The listing builds one solid part. Answer for the finished solid, in the listing's coordinates (mm). A direction names the side the tool comes from. Give positions to 0.01 mm unless a question says otherwise; leave off trailing zeros. Loops run counter-clockwise (first coordinate to the right, second up) from the corner with the lowest first, then second, coordinate; pieces in that order, holes last. Notation, with made-up numbers: (22.25, 30.25) - (32.25, 30.25) arc R24 cw to (32.25, 63.25) - close; hole circle Ø8 at (33, 9.5). An arc over 180 degrees is marked (long way). Write item = value, one per line. Start each with the question number.
1) The part is cut by section B-B on y = -5. Write down the section's boundary in (x, z).
2) The mould has two halves that part along Y. Classify faces 1 (the cylindrical face through (-4.385, 2.465, 2.895)), 2 (the flat face through (-6, -5.5, 6)), 3 (the flat face through (-13, 0, 13)): +Y half, -Y half, draft (parallel to the pull), parting line (faces both ways), or undercut.
3) The part is cut by section A-A on x = -21.5. Write down the section's boundary in (y, z).
4) A flat-ended cylindrical pin translates along its axis: P1, Ø1, axis at x = -15, z = 9, coming from the +Y side. Find the tip coordinate at first contact, or state that the pin passes through.
5) The part is cut by section D-D on y = 1.5. Write down the section's boundary in (x, z).
6) Which of the six approach directions +Z, -Z, +X, -X, +Y, -Y give full straight-line access (tool end or side, diameter ignored) to faces 4 (the flat face through (-19, 5, 19)), 5 (the cylindrical face through (-6.46, 2.46, 22.47)), 6 (the flat face through (-20, -5.5, 20))?
7) Consider probe 1 along X at (y, z) = (-3.7, 19.5); probe 2 along Z at (x, y) = (-19.5, -3.45); probe 3 along Y at (x, z) = (-19, 17.5). Determine where each line is inside the solid, lowest interval first.
8) The part is cut by section C-C on z = 21.75. Write down the section's boundary in (x, y), plus the area to 3 significant figures.
from build123d import *

# Parameters (mm, degrees)
F0_W      = 25
F0_H      = 25
F1_DEPTH  = 10
F2_R      = 3.5
F3_DEPTH  = 5
F4_R      = 4
F1_FACE_W = 25
F1_FACE_H = 25
F5_DEPTH  = 5.5


with BuildPart() as f1:
    # F0 (on Front) → F1 (new body)
    with BuildSketch(Plane.XZ):
        with Locations((-12.5, 12.5)):
            Rectangle(F0_W, F0_H)
    extrude(amount=F1_DEPTH)

    # F2 (on Front) → F3 (join)
    with BuildSketch(Plane.XZ):
        with Locations((-19, 19)):
            Circle(F2_R)
        with Locations((-19, 6)):
            Circle(F2_R)
        with Locations((-6, 6)):
            Circle(F2_R)
        with Locations((-6, 19)):
            Circle(F2_R)
    extrude(amount=-F3_DEPTH)

    # F4 (on Front) + F1_face (on face) → F5 (cut)
    with BuildSketch(Plane.XZ):
        with Locations((-19.5, 19.5)):
            Circle(F4_R)
        with Locations((-19.5, 5.5)):
            Circle(F4_R)
        with Locations((-5.5, 5.5)):
            Circle(F4_R)
        with Locations((-5.5, 19.5)):
            Circle(F4_R)
    with BuildSketch(Plane(origin=(-12.5, -10, 12.5), x_dir=(1, 0, 0), z_dir=(0, -1, 0))):
        Rectangle(F1_FACE_W, F1_FACE_H)
    extrude(amount=F5_DEPTH, mode=Mode.SUBTRACT)


solid = f1.part
Answer below:
q1.outline = (-25, 0) - (0, 0) - (0, 25) - (-25, 25) - close; hole circle Ø8 at (-19.5, 5.5); hole circle Ø8 at (-19.5, 19.5); hole circle Ø8 at (-5.5, 5.5); hole circle Ø8 at (-5.5, 19.5)
q2.face_1 = draft
q2.face_2 = undercut
q2.face_3 = +Y half
q3.outline = (-10, 0) - (0, 0) - (0, 2.04) - (-5.5, 2.04) - (-5.5, 8.96) - (0, 8.96) - (0, 16.04) - (-5.5, 16.04) - (-5.5, 22.96) - (0, 22.96) - (0, 25) - (-10, 25) - close; (0, 3.55) - (5, 3.55) - (5, 8.45) - (0, 8.45) - close; (0, 16.55) - (5, 16.55) - (5, 21.45) - (0, 21.45) - close
q4.P1 = 0
q5.outline = circle Ø7 at (-19, 6); circle Ø7 at (-19, 19); circle Ø7 at (-6, 6); circle Ø7 at (-6, 19)
q6.face_4 = +Z, -Z, +X, -X, +Y
q6.face_5 = +Y
q6.face_6 = none
q7.probe_1 = -25 to -23.5, -15.5 to -9.5, -1.5 to 0
q7.probe_2 = 0 to 1.5, 9.5 to 15.5, 23.5 to 25
q7.probe_3 = -10 to -5.5, 0 to 5
q8.outline = (-25, -10) - (0, -10) - (0, 0) - (-2.19, 0) - (-2.19, -5.5) - (-8.81, -5.5) - (-8.81, 0) - (-16.19, 0) - (-16.19, -5.5) - (-22.81, -5.5) - (-22.81, 0) - (-25, 0) - close; (-21.17, 0) - (-16.83, 0) - (-16.83, 5) - (-21.17, 5) - close; (-8.17, 0) - (-3.83, 0) - (-3.83, 5) - (-8.17, 5) - close
q8.area = 221 mm2
